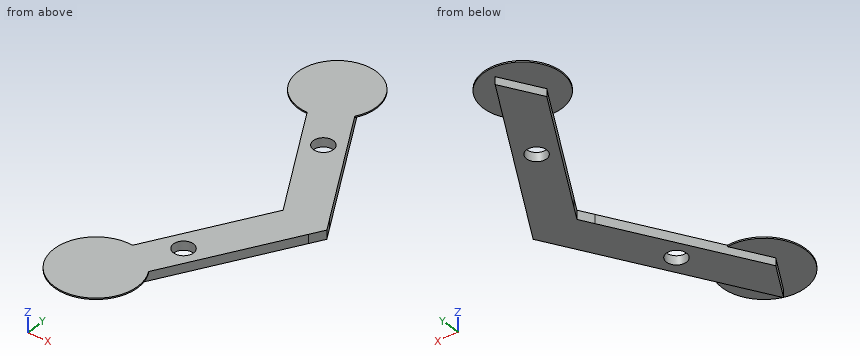
Autodesk Inventor part; units mm, degrees
ref_plane "YZ Plane" through (0, 0, 0) normal (1, 0, 0) x (0, 1, 0)
ref_plane "XZ Plane" through (0, 0, 0) normal (0, 1, 0) x (-1, 0, 0)
ref_plane "XY Plane" through (0, 0, 0) normal (0, 0, 1) x (1, 0, 0)
sketch "Sketch1" plane through (0, 0, 0) normal (0, 0, 1) x (1, 0, 0)
  circle A0 centre (0, 0) radius 7.5
  line L0 (-21.2869, 0) -> (22.3896, 0) construction
  line L1 (0, 21.9302) -> (0, -69.0741) construction
  line L2 (24.9778, -67) -> (-24.9778, -67) construction
  line L3 (-17.5, -57) -> (17.5, -57)
  line L4 (17.5, -57) -> (17.5, -67)
  line L5 (17.5, -67) -> (-17.5, -67)
  line L6 (-17.5, -67) -> (-17.5, -57)
  line L7 (-37.5278, -67) -> (-18.5, -67)
  line L8 (-18.5, -67) -> (-18.5, -56)
  line L9 (-17.5, -62) -> (17.5, -62) construction
  line L10 (-18.5, -59) -> (-22.5, -59)
  line L11 (-22.5, -59) -> (-22.5, -65)
  line L12 (-22.5, -65) -> (-18.5, -65)
  line L13 (-18.5, -65) -> (-18.5, -59)
  line L14 (-17.5, -60) -> (-21.5, -60)
  line L15 (-21.5, -60) -> (-21.5, -64)
  line L16 (-21.5, -64) -> (-17.5, -64)
  line L17 (-17.5, -64) -> (-17.5, -60)
  line L18 (-18.5, -56) -> (-28.8675, -56)
  line L19 (17.5, -60) -> (21.5, -60)
  line L20 (21.5, -60) -> (21.5, -64)
  line L21 (21.5, -64) -> (17.5, -64)
  line L22 (17.5, -64) -> (17.5, -60)
  line L23 (18.5, -67) -> (18.5, -56)
  line L24 (18.5, -67) -> (37.5278, -67)
  line L25 (18.5, -65) -> (22.5, -65)
  line L26 (22.5, -65) -> (22.5, -59)
  line L27 (22.5, -59) -> (18.5, -59)
  line L28 (18.5, -59) -> (18.5, -65)
  line L29 (18.5, -56) -> (28.8675, -56)
  line L30 (-23.7704, -40) -> (28.6931, -40) construction
  line L31 (-17.1762, -35.75) -> (17.1762, -35.75)
  line L32 (-22.0836, -44.25) -> (22.0836, -44.25)
  circle A1 centre (0, -40) radius 2.25
  line L33 (-7.5, -16) -> (7.5, -16)
  line L34 (7.5, -16) -> (7.5, -21)
  line L35 (7.5, -26) -> (-7.5, -26)
  line L36 (-7.5, -26) -> (-7.5, -24)
  line L37 (7.5, -21) -> (-7.5, -21) construction
  line L38 (-7.5, -18) -> (-3.5, -18)
  line L39 (-3.5, -18) -> (-3.5, -21)
  line L40 (-3.5, -24) -> (-7.5, -24)
  line L41 (-7.5, -24) -> (-7.5, -23)
  line L42 (-8.5, -19) -> (-4.5, -19)
  line L43 (-4.5, -19) -> (-4.5, -23)
  line L44 (-4.5, -23) -> (-8.5, -23)
  line L45 (-8.5, -23) -> (-8.5, -19)
  line L46 (7.5, -18) -> (3.5, -18)
  line L47 (3.5, -18) -> (3.5, -21)
  line L48 (3.5, -24) -> (7.5, -24)
  line L49 (7.5, -24) -> (7.5, -18)
  line L50 (8.5, -19) -> (4.5, -19)
  line L51 (4.5, -19) -> (4.5, -23)
  line L52 (4.5, -23) -> (8.5, -23)
  line L53 (8.5, -23) -> (8.5, -19)
  line L54 (-9.815, -19) -> (-31.1769, -56)
  line L55 (-7.5056, -19) -> (-28.8675, -56)
  line L56 (7.5056, -19) -> (28.8675, -56)
  line L57 (-4.5, -21) -> (-8.5, -21)
  line L58 (4.5, -21) -> (8.5, -21)
  line L59 (-21.5, -62) -> (-17.5, -62)
  line L60 (17.5, -62) -> (21.5, -62)
  line L61 (-22.5, -62) -> (-18.5, -62)
  line L62 (22.5, -62) -> (18.5, -62)
  line L63 (-7.5, -21) -> (-3.5, -21)
  line L64 (3.5, -21) -> (7.5, -21)
  line L65 (-28.8675, -56) -> (-31.1769, -56)
  line L66 (28.8675, -56) -> (31.1769, -56)
  line L67 (-10.8853, -24.8539) -> (-12.6173, -23.8539)
  line L68 (10.8875, -24.8576) -> (12.6195, -23.8576)
  line L69 (7.5, -23) -> (7.5, -24)
  line L70 (-7.5, -23) -> (-7.5, -21)
  line L71 (-7.5, -24) -> (-7.5, -16)
  line L72 (7.5, -24) -> (7.5, -26)
  line L73 (-7.5, -21) -> (-7.5, -18)
  line L74 (-3.5, -21) -> (-3.5, -24)
  line L75 (3.5, -21) -> (3.5, -24)
  line L76 (7.5, -21) -> (7.5, -23)
  line L77 (-18.4752, 0) -> (-9.2376, 16)
  line L78 (-9.2376, 16) -> (9.2376, 16)
  line L79 (9.2376, 16) -> (18.4752, 0)
  line L80 (18.4752, 0) -> (9.2376, -16)
  line L81 (9.2376, -16) -> (-9.2376, -16)
  line L82 (-9.2376, -16) -> (-18.4752, 0)
  line L83 (-77.3649, 0) -> (-38.6825, 67) construction
  line L84 (-38.6825, 67) -> (38.6825, 67) construction
  line L85 (38.6825, 67) -> (77.3649, 0) construction
  line L86 (77.3649, 0) -> (38.6825, -67) construction
  line L87 (38.6825, -67) -> (-38.6825, -67) construction
  line L88 (-38.6825, -67) -> (-77.3649, 0) construction
  line L89 (-9.2376, -16) -> (-38.6825, -67) construction
  line L90 (9.2376, -16) -> (38.6825, -67) construction
  line L91 (0, -16.7974) -> (0, -26) construction
  line L92 (9.815, -19) -> (31.1769, -56)
  line L93 (-8.5, -19) -> (-9.815, -19)
  line L94 (8.5, -19) -> (9.815, -19)
  line L95 (-8.5, -23) -> (-9.815, -23)
  line L96 (8.5, -23) -> (9.815, -23)
  line L97 (-31.1769, -56) -> (-37.5278, -67)
  line L98 (31.1769, -56) -> (37.5278, -67)
  circle A2 centre (12.25, 0) radius 2.25
  circle A3 centre (6.125, 10.6088) radius 2.25
  circle A4 centre (-6.125, 10.6088) radius 2.25
  circle A5 centre (-12.25, 0) radius 2.25
  circle A6 centre (-6.125, -10.6088) radius 2.25
  circle A7 centre (6.125, -10.6088) radius 2.25
  line L99 (22.3723, -32.75) -> (39.5485, -3)
  line L100 (27.2798, -41.25) -> (49.3634, -3)
  circle A8 centre (34.641, -20) radius 2.25
  line L101 (39.5485, 3) -> (22.3723, 32.75)
  line L102 (49.3634, 3) -> (27.2798, 41.25)
  circle A9 centre (34.641, 20) radius 2.25
  line L103 (17.1762, 35.75) -> (-17.1762, 35.75)
  line L104 (22.0836, 44.25) -> (-22.0836, 44.25)
  circle A10 centre (0, 40) radius 2.25
  line L105 (-22.3723, 32.75) -> (-39.5485, 3)
  line L106 (-27.2798, 41.25) -> (-49.3634, 3)
  circle A11 centre (-34.641, 20) radius 2.25
  line L107 (-39.5485, -3) -> (-22.3723, -32.75)
  line L108 (-49.3634, -3) -> (-27.2798, -41.25)
  circle A12 centre (-34.641, -20) radius 2.25
  line L109 (22.3723, -32.75) -> (27.2798, -41.25)
  line L110 (49.3634, -3) -> (51.0955, 0)
  line L111 (49.3634, 3) -> (51.0955, 0)
  line L112 (39.5485, -3) -> (41.2805, 0)
  line L113 (39.5485, 3) -> (41.2805, 0)
  line L114 (7.3612, 4.25) -> (38.8268, 4.25)
  line L115 (7.3612, -4.25) -> (38.8268, -4.25)
  arc A13 (8.5, 0) -> (7.3612, 4.25) centre (0, 0) ccw
  arc A14 (7.3612, -4.25) -> (8.5, 0) centre (0, 0) ccw
  arc A15 (7.3612, 4.25) -> (7.3612, -4.25) centre (0, 0) ccw
  line L116 (22.3723, 32.75) -> (27.2798, 41.25)
  circle A16 centre (26.0807, 34.891) radius 8.782
  circle A17 centre (26.0807, -34.1103) radius 9.356
  point P0 (0, -57)
  point P1 (0, -67)
  point P2 (0, -62)
  point P3 (0, -21)
  dimension "d0" = 15
  dimension "d16" = 10
  dimension "d20" = 6
  dimension "d21" = 4
  dimension "d22" = 4
  dimension "d23" = 1
  dimension "d24" = 1
  dimension "d25" = 35
  dimension "d27" = 3
  dimension "d28" = 4
  dimension "d29" = 1
  dimension "d30" = 6
  dimension "d31" = 4
  dimension "d32" = 1
  dimension "d34" = 3
  dimension "d35" = 27
  dimension "d39" = 4.5
  dimension "d41" = 2
  dimension "d42" = 2
  dimension "d44" = 10
  dimension "d45" = 4
  dimension "d46" = 6
  dimension "d48" = 4
  dimension "d49" = 1
  dimension "d50" = 4
  dimension "d52" = 6
  dimension "d53" = 4
  dimension "d54" = 4
  dimension "d55" = 1
  dimension "d56" = 4
  dimension "d57" = 15
  dimension "d60" = 2
  dimension "d81" = 16
  dimension "d83" = 67
  dimension "d84" = 1
  dimension "d86" = 2
  dimension "d87" = 1
  dimension "d88" = 5
  dimension "d89" = 3
  dimension "d90" = 3
  dimension "d112" = 4.5
  dimension "d113" = 2.5
  dimension "d116" = 360
  dimension "d120" = 360
  dimension "d122" = 2
  dimension "d123" = 2
  dimension "d124" = 1
extrude "Extrusion8" add sketch "Sketch1" against normal blind 2 contours A17 L100 L109 L99 | L99 L112 L113 L101 A16 L102 L111 L110 L100 A17 | A16 L101 L116 L102 picked at (27.7457, 34.7764)
extrude "Extrusion9" add sketch "Sketch1" against normal blind 0.3 contours A17 L31 L56 | L56 A17 L92 | L92 A17 L99 L109 L100 | A17 L56 L31 | A17 L100 L109 L99 | A16 L101 L116 L102 | L102 L116 L101 A16
equation "\"d20\" = hinge_w"
equation "\"d21\" = hinge_d"
equation "\"d22\" = hinge_w - 2 * hinge_sp"
equation "\"d23\" = hinge_sp"
equation "\"d24\" = sp"
equation "\"d28\" = hinge_w - 2 * hinge_sp"
equation "\"d29\" = sp"
equation "\"d30\" = hinge_w"
equation "\"d31\" = hinge_d"
equation "\"d32\" = hinge_sp"
equation "\"d39\" = screw"
equation "\"d45\" = hinge_d"
equation "\"d46\" = hinge_w"
equation "\"d48\" = hinge_d"
equation "\"d49\" = hinge_sp"
equation "\"d50\" = hinge_w - 2 * hinge_sp"
equation "\"screw\" = 4.5"
equation "\"k\" = 0.4"
equation "\"sp\" = 1"
equation "\"d14\" = sp"
equation "\"d15\" = sp"
equation "\"d19\" = sp"
equation "\"hinge_d\" = 4"
equation "\"hinge_w\" = 6"
equation "\"hinge_sp\" = 1"
properties part number "RobotBase" material "Glass"
Can you work these out from the model? Positions are in its coordinate system, mm. Coordinates: 2 decimals unless noted, no trailing zeros. Loops run counter-clockwise (first coordinate to the right, second up) from the corner with the lowest first, then second, coordinate; pieces in that order, holes last. Notation, with made-up numbers: (61.25, 4) - (115.25, 4) arc R11 cw to (115.25, 14) - close; hole circle Ø1 at (-13.5, 16). An arc over 180 degrees is marked (long way). Put each result on its own line as item: value. Start each with the question number.
Item 1: If I drill on line 1 along Y through (x, z) = (32, -0.5); line 2 along X through (y, z) = (-19, -1.5); line 3 along Y through (x, z) = (26.5, -0.8), over which ranges is the centre line in solid material (lowest first)?
Item 2: Suppose I cut it at D-D (y = -21.5). Please give me the cut outline in (x, z), and give its area (3 significant figures).
Item 3: Suppose I cut it at C-C (x = 29.5). Please give me the cut outline in (y, z), and give its area (3 significant figures).
Item 4: For pin 1 (10 mm diameter, centred on x = 45.5, y = 22, fed in from -Z); pin 2 (6 mm diameter, centred on x = 21, y = -23, fed in from -Z), each with a flat end and sliding along its axis, tell me the tip position at first contact or that it passes through.
Item 5: Suppose I cut it at B-B (y = 21). Please give me the cut outline in (x, z).
Item 6: Suppose I cut it at A-A (z = -1.15). Please give me the cut outline in (x, y), and give its area (3 significant figures).
Here are the results:
1. line 1: -33.07 to -16.07, 16.07 to 33.07
1. line 2: 30.31 to 32.63, 36.66 to 40.13
1. line 3: -39.9 to -25.6, 25.6 to 39.9
2. outline: (28.87, -2) - (32.96, -2) - (32.96, 0) - (28.87, 0) - close; (36.32, -2) - (38.68, -2) - (38.68, 0) - (36.32, 0) - close
2. area: 12.9 mm²
3. outline: (-42.82, -0.3) - (-37.4, -0.3) - (-37.4, -2) - (-20.4, -2) - (-20.4, 0) - (-42.82, 0) - close; (20.4, -2) - (37.4, -2) - (37.4, -0.3) - (42.98, -0.3) - (42.98, 0) - (20.4, 0) - close
3. area: 71.3 mm²
4. pin 1: through
4. pin 2: z = -0.3
5. outline: (29.16, -2) - (32.63, -2) - (32.63, 0) - (29.16, 0) - close; (36.66, -2) - (38.97, -2) - (38.97, 0) - (36.66, 0) - close
6. outline: (22.37, -32.75) - (27.28, -41.25) - (49.36, -3) - (51.1, 0) - (49.36, 3) - (27.28, 41.25) - (22.37, 32.75) - (39.55, 3) - (41.28, 0) - (39.55, -3) - close; hole circle Ø4.5 at (34.64, -20); hole circle Ø4.5 at (34.64, 20)
6. area: 694 mm²
